from build123d import *

# Parameters (mm, degrees)
SKETCH2_R       = 3.25
F_6_5_HUL_DEPTH = 25


with BuildPart() as part:
    # Sketch1 → Base-Revolve (revolve)
    with BuildSketch(Plane.XY):
        with BuildLine():
            Line((1, 14), (95, 14))
            ThreePointArc((95, 14), (96.060660172, 13.560660172), (96.5, 12.5))
            Line((96.5, 12.5), (96.5, 11.7))
            ThreePointArc((96.5, 11.7), (96.939339828, 10.639339828), (98, 10.2))
            Line((98, 10.2), (102.5, 10.2))
            Line((102.5, 10.2), (105.617691454, 12))
            Line((105.617691454, 12), (127.5, 12))
            Line((127.5, 12), (129.5, 10))
            Line((129.5, 10), (129.5, 0))
            Line((129.5, 0), (0, 0))
            Line((0, 0), (0, 13))
            ThreePointArc((0, 13), (0.292893219, 13.707106781), (1, 14))
        make_face()
    revolve(axis=Axis((-12.994157099, 0, 0), (1, 0, 0)))

    # Sketch2 → ø6.5 hul (cut, symmetric)
    with BuildSketch(Plane.XY):
        with Locations((122, 0)):
            Circle(SKETCH2_R)
    extrude(amount=F_6_5_HUL_DEPTH, both=True, mode=Mode.SUBTRACT)


solid = part.part
Input: part model. Units: mm. Frame: model coordinates. A direction names the side the tool comes from. Coordinates: 2 decimals unless noted, no trailing zeros. Loops run counter-clockwise (first coordinate to the right, second up) from the corner with the lowest first, then second, coordinate; pieces in that order, holes last.
Q1. Set-up query: faces 1 (the face through (116.712, 5.537, -10.646)), 2 (the face through (102.7, 9.84, 3.1)), 3 (the face through (48.658, 12.932, -5.362)). Return all of +Z, -Z, +X, -X, +Y, -Y with unobstructed straight access to the full face (end or side cutting, diameter ignored); none if empty.
Q2. Contact query for flat-ended pins moving along their axis: pin 1 (1.5 mm diameter, centred on x = 94.5, z = 9, fed in from -Y); pin 2 (1.5 mm diameter, centred on y = 11, z = 0, fed in from -X); pin 3 (6 mm diameter, centred on x = 24, z = -3.5, fed in from +Y); pin 4 (3 mm diameter, centred on x = 65.5, z = -5, fed in from +Y). Output: stop coordinate, or through.
Q3. Cut plane B-B (z = 0). Output: boundary loops of the cut face in (x, y), then the cut area to 3 significant figures.
Q4. Cut plane C-C (x = 67). Output: boundary loops of the cut face in (y, z), then the cut area to 3 significant figures.
Q5. Draft query along X for faces 4 (the face through (125.1, 0.98, 0.17)), 5 (the face through (0, 0, 0)), 6 (the face through (129.5, 0, 0)). Return one class per face: +X half, -X half, draft (parallel to the pull), parting line (faces both ways), or undercut.
Q6. Material intervals for line 1 (X direction, y = 0, z = 6.75); line 2 (Z direction, x = 111, y = 0.5), sorted ascending.
Q7. Cut plane A-A (y = 0). Output: boundary loops of the cut face in (x, z), then the cut area to 3 significant figures.
Q8. Cut plane D-D (x = 122). Output: boundary loops of the cut face in (y, z).
Working result:
1. face 1: +X
1. face 2: none
1. face 3: +X, -X
2. pin 1: stops at y = -11.31
2. pin 2: stops at x = 0
2. pin 3: stops at y = 13.99
2. pin 4: stops at y = 13.56
3. outline: (0, -13) arc R1 ccw to (1, -14) - (95, -14) arc R1.5 ccw to (96.5, -12.5) - (96.5, -11.7) arc R1.5 cw to (98, -10.2) - (102.5, -10.2) - (105.62, -12) - (127.5, -12) - (129.5, -10) - (129.5, 10) - (127.5, 12) - (105.62, 12) - (102.5, 10.2) - (98, 10.2) arc R1.5 cw to (96.5, 11.7) - (96.5, 12.5) arc R1.5 ccw to (95, 14) - (1, 14) arc R1 ccw to (0, 13) - close; hole circle Ø6.5 at (122, 0)
3. area: 3,430 mm2
4. outline: circle Ø28 at (0, 0)
4. area: 616 mm2
5. face 4: undercut
5. face 5: -X half
5. face 6: +X half
6. line 1: x = 0 to 118.75, 125.25 to 129.5
6. line 2: z = -11.99 to 11.99
7. outline: (0, -13) arc R1 ccw to (1, -14) - (95, -14) arc R1.5 ccw to (96.5, -12.5) - (96.5, -11.7) arc R1.5 cw to (98, -10.2) - (102.5, -10.2) - (105.62, -12) - (118.75, -12) - (118.75, 12) - (105.62, 12) - (102.5, 10.2) - (98, 10.2) arc R1.5 cw to (96.5, 11.7) - (96.5, 12.5) arc R1.5 ccw to (95, 14) - (1, 14) arc R1 ccw to (0, 13) - close; (125.25, -12) - (127.5, -12) - (129.5, -10) - (129.5, 10) - (127.5, 12) - (125.25, 12) - close
7. area: 3,310 mm2
8. outline: (-3.25, -11.55) - (-3.25, 11.55) arc R12 ccw to start; (3.25, -11.55) arc R12 ccw to (3.25, 11.55) - close
